Geometry check sheet. Reference: the model listing, model coordinates, mm. A direction names the side the tool comes from. Round coordinates to 2 decimals unless told otherwise and drop trailing zeros. Write each loop counter-clockwise with the first axis right and the second up, starting at its lowest first coordinate (ties: lowest second). Pieces come first, ordered by that corner, then holes. Notation, with made-up numbers: M -19.5,43.5 L 32.5,43.5 A18 ccw 32.5,60.5 Z; hole C -4,8.5 d5. An arc over 180 degrees is marked long. Use a Markdown table: item, result.
Autodesk Inventor part; units mm, degrees
ref_plane "YZ Plane" through (0, 0, 0) normal (1, 0, 0) x (0, 1, 0)
ref_plane "XZ Plane" through (0, 0, 0) normal (0, 1, 0) x (-1, 0, 0)
ref_plane "XY Plane" through (0, 0, 0) normal (0, 0, 1) x (1, 0, 0)
sketch "Sketch1" plane through (0, 0, 0) normal (0, 0, 1) x (1, 0, 0)
  line L0 (50, -50) -> (-50, -50)
  line L1 (-50, -50) -> (-50, 50)
  line L2 (-50, 50) -> (50, 50)
  line L3 (50, 50) -> (50, -50)
  line L4 (50, -50) -> (-50, 50) construction
  line L5 (-50, -50) -> (50, 50) construction
  line L6 (-50, -41.5) -> (-56.5, -41.5)
  line L7 (-56.5, -41.5) -> (-56.5, 41.5)
  line L8 (-56.5, 41.5) -> (-50, 41.5)
  line L9 (-50, 41.5) -> (-50, -41.5)
  line L10 (-41.5, 50) -> (41.5, 50)
  line L11 (41.5, 50) -> (41.5, 56.5)
  line L12 (41.5, 56.5) -> (-41.5, 56.5)
  line L13 (-41.5, 56.5) -> (-41.5, 50)
  line L14 (50, 41.5) -> (56.5, 41.5)
  line L15 (56.5, 41.5) -> (56.5, -41.5)
  line L16 (56.5, -41.5) -> (50, -41.5)
  line L17 (50, -41.5) -> (50, 41.5)
  line L18 (41.5, -50) -> (-41.5, -50)
  line L19 (-41.5, -50) -> (-41.5, -56.5)
  line L20 (-41.5, -56.5) -> (41.5, -56.5)
  line L21 (41.5, -56.5) -> (41.5, -50)
  point P0 (0, 0)
  point P1 (-50, 0)
  point P2 (0, 50)
  point P3 (50, 0)
  point P4 (0, -50)
  dimension "d0" = 100
  dimension "d1" = 6.5
  dimension "d2" = 8.5
extrude "Extrusion1" add sketch "Sketch1" along normal blind 57 and the other way blind 56.5
sketch "Sketch2" plane through (0, 0, 57) normal (0, 0, 1) x (1, 0, 0)
  line L0 (-41.5, -50) -> (-41.5, -56.5)
  line L1 (-41.5, -56.5) -> (41.5, -56.5)
  line L2 (41.5, -56.5) -> (41.5, -50)
  line L3 (41.5, -50) -> (50, -50)
  line L4 (50, -50) -> (50, -41.5)
  line L5 (50, -41.5) -> (56.5, -41.5)
  line L6 (56.5, -41.5) -> (56.5, 41.5)
  line L7 (56.5, 41.5) -> (50, 41.5)
  line L8 (50, 41.5) -> (50, 50)
  line L9 (50, 50) -> (41.5, 50)
  line L10 (41.5, 50) -> (41.5, 56.5)
  line L11 (41.5, 56.5) -> (-41.5, 56.5)
  line L12 (-41.5, 56.5) -> (-41.5, 50)
  line L13 (-41.5, 50) -> (-50, 50)
  line L14 (-50, 50) -> (-50, 41.5)
  line L15 (-50, 41.5) -> (-56.5, 41.5)
  line L16 (-56.5, 41.5) -> (-56.5, -41.5)
  line L17 (-56.5, -41.5) -> (-50, -41.5)
  line L18 (-50, -41.5) -> (-50, -50)
  line L19 (-50, -50) -> (-41.5, -50)
  line L20 (-50, -41.5) -> (-50, -50)
  line L21 (-50, -41.5) -> (-41.5, -41.5)
  line L22 (-41.5, -41.5) -> (-41.5, -50)
  line L23 (-50, 50) -> (-50, 41.5)
  line L24 (-50, 41.5) -> (-41.5, 41.5)
  line L25 (-41.5, 41.5) -> (-41.5, 50)
  line L26 (41.5, 56.5) -> (41.5, 50)
  line L27 (41.5, 50) -> (41.5, 41.5)
  line L28 (41.5, 41.5) -> (50, 41.5)
  line L29 (41.5, -50) -> (41.5, -41.5)
  line L30 (50, -41.5) -> (56.5, -41.5)
  line L31 (50, -41.5) -> (41.5, -41.5)
  point P0 (0, 0)
extrude "Extrusion2" cut sketch "Sketch2" against normal blind 1 contours L22 L21 L17 L16 L15 L24 L25 L12 L11 L10 L27 L28 L7 L6 L5 L31 L29 L2 L1 L0
sketch "Sketch3" plane through (56.5, -41.5, -56.5) normal (1, 0, 0) x (0, 0, -1)
  line L0 (-112.5, 83) -> (-112.5, 0)
  line L1 (0, 0) -> (-112.5, 0)
  line L2 (0, 83) -> (0, 0)
  line L3 (0, 83) -> (-112.5, 83)
  line L4 (-86.5, 5.25) -> (0, 5.25)
  line L5 (0, 5.25) -> (0, 77.75)
  line L6 (0, 77.75) -> (-86.5, 77.75)
  line L7 (-86.5, 77.75) -> (-86.5, 5.25)
  line L8 (0, 83) -> (0, 0)
  point P0 (-56.5, 41.5)
  point P1 (0, 41.5)
  dimension "d9" = 72.5
  dimension "d10" = 86.5
split_face "Split1"
sketch "Sketch4" plane through (0, 0, -56.5) normal (0, 0, -1) x (-1, 0, 0)
  line L0 (41.5, -56.5) -> (41.5, -50)
  line L1 (-41.5, -56.5) -> (41.5, -56.5)
  line L2 (-41.5, -50) -> (-41.5, -56.5)
  line L3 (-41.5, -41.5) -> (-41.5, -50)
  line L4 (-50, -41.5) -> (-41.5, -41.5)
  line L5 (-56.5, -41.5) -> (-50, -41.5)
  line L6 (-56.5, 41.5) -> (-56.5, -41.5)
  line L7 (-50, 41.5) -> (-56.5, 41.5)
  line L8 (-41.5, 41.5) -> (-50, 41.5)
  line L9 (-41.5, 50) -> (-41.5, 41.5)
  line L10 (-41.5, 56.5) -> (-41.5, 50)
  line L11 (41.5, 56.5) -> (-41.5, 56.5)
  line L12 (41.5, 50) -> (41.5, 56.5)
  line L13 (41.5, 41.5) -> (41.5, 50)
  line L14 (50, 41.5) -> (41.5, 41.5)
  line L15 (56.5, 41.5) -> (50, 41.5)
  line L16 (56.5, -41.5) -> (56.5, 41.5)
  line L17 (50, -41.5) -> (56.5, -41.5)
  line L18 (41.5, -41.5) -> (50, -41.5)
  line L19 (41.5, -50) -> (41.5, -41.5)
  point P0 (0, 0)
split_face "Split2"
properties part number "CubeSatStandard" material "Aluminum 6061"
Item 1: Cross-section at A-A, the plane y = 47. Record the cut outline in (x, z), and give its area (3 significant figures).
Outcome:
| item | result |
|---|---|
| outline | M -50,-56.5 L 50,-56.5 L 50,57 L 41.5,57 L 41.5,56 L -41.5,56 L -41.5,57 L -50,57 Z |
| area | 11,300 mm2 |
Item 2: Material ranges on line 1 along Z through (x, y) = (19, 22.5); line 2 along X through (y, z) = (-42, 25.5), recorded low to high. Write a range as from..to.
Outcome:
| item | result |
|---|---|
| line 1 | z = -56.5..56 |
| line 2 | x = -50..50 |
Item 3: Cross-section at B-B, the plane z = 26. Record the cut outline in (x, y), and give its area (3 significant figures).
Outcome:
| item | result |
|---|---|
| outline | M -56.5,-41.5 L -50,-41.5 L -50,-50 L -41.5,-50 L -41.5,-56.5 L 41.5,-56.5 L 41.5,-50 L 50,-50 L 50,-41.5 L 56.5,-41.5 L 56.5,41.5 L 50,41.5 L 50,50 L 41.5,50 L 41.5,56.5 L -41.5,56.5 L -41.5,50 L -50,50 L -50,41.5 L -56.5,41.5 Z |
| area | 12,200 mm2 |
Item 4: Go/stop test with flat-tipped pins: pin 1 (3 mm diameter, centred on x = -3.5, y = 17, fed in from +Z); pin 2 (9.5 mm diameter, centred on x = -48, z = 26, fed in from -Y); pin 3 (3 mm diameter, centred on x = -54, z = -8, fed in from -Y). Record where each tip stops, or that it passes through.
Outcome:
| item | result |
|---|---|
| pin 1 | stops at z = 56 |
| pin 2 | stops at y = -50 |
| pin 3 | stops at y = -41.5 |
Item 5: Access from +Z, -Z, +X, -X, +Y, -Y to the whole of each face (thin tool, end or side, straight path). Record for faces 1 (the face through (50, 46, -1)), 2 (the face through (-41.5, -53, -1)), 3 (the face through (-46, 50, -1)), 4 (the face through (50, -46, -1)).
Outcome:
| item | result |
|---|---|
| face 1 | +Z, -Z, +X, +Y |
| face 2 | +Z, -Z, -X, -Y |
| face 3 | +Z, -Z, -X, +Y |
| face 4 | +Z, -Z, +X, -Y |
